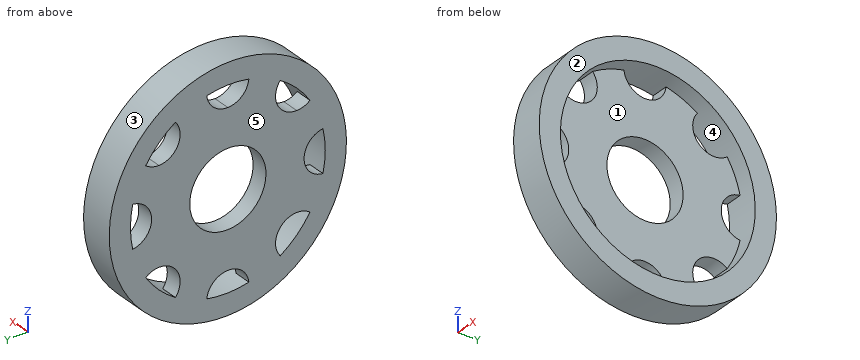
from build123d import *

# Parameters (mm, degrees)
ESBO_O1_R                = 4.5
RESSALTO_EXTRUS_O1_DEPTH = 2
ESBO_O2_R                = 14
ESBO_O2_R_2              = 11.5
RESSALTO_EXTRUS_O2_DEPTH = 2


with BuildPart() as part:
    # Esboço1 → Ressalto-extrusão1 (new body)
    with BuildSketch(Plane(origin=(0, 0, 0), x_dir=(0, 0, -1), z_dir=(1, 0, 0))):
        with BuildLine():
            ThreePointArc((11.22826087, -2.485187688), (9, 0), (11.22826087, 2.485187688))
            ThreePointArc((11.22826087, 2.485187688), (10.624614624, 4.400859472), (9.696872469, 6.182286335))
            ThreePointArc((9.696872469, 6.182286335), (6.363961031, 6.363961031), (6.182286335, 9.696872469))
            ThreePointArc((6.182286335, 9.696872469), (4.400859472, 10.624614624), (2.485187688, 11.22826087))
            ThreePointArc((2.485187688, 11.22826087), (0, 9), (-2.485187688, 11.22826087))
            ThreePointArc((-2.485187688, 11.22826087), (-4.400859472, 10.624614624), (-6.182286335, 9.696872469))
            ThreePointArc((-6.182286335, 9.696872469), (-5.773380668, 8.961304948), (-5.631727984, 8.131727984))
            ThreePointArc((-5.631727984, 8.131727984), (-7.050724101, 5.877525108), (-9.696872469, 6.182286335))
            ThreePointArc((-9.696872469, 6.182286335), (-10.624614624, 4.400859472), (-11.22826087, 2.485187688))
            ThreePointArc((-11.22826087, 2.485187688), (-9.638636545, 1.668929623), (-9, 0))
            ThreePointArc((-9, 0), (-9.638636545, -1.668929623), (-11.22826087, -2.485187688))
            ThreePointArc((-11.22826087, -2.485187688), (-10.624614624, -4.400859472), (-9.696872469, -6.182286335))
            ThreePointArc((-9.696872469, -6.182286335), (-7.050724101, -5.877525108), (-5.631727984, -8.131727984))
            ThreePointArc((-5.631727984, -8.131727984), (-5.773380668, -8.961304948), (-6.182286335, -9.696872469))
            ThreePointArc((-6.182286335, -9.696872469), (-4.400859472, -10.624614624), (-2.485187688, -11.22826087))
            ThreePointArc((-2.485187688, -11.22826087), (0, -9), (2.485187688, -11.22826087))
            ThreePointArc((2.485187688, -11.22826087), (4.400859472, -10.624614624), (6.182286335, -9.696872469))
            ThreePointArc((6.182286335, -9.696872469), (6.363961031, -6.363961031), (9.696872469, -6.182286335))
            ThreePointArc((9.696872469, -6.182286335), (10.624614624, -4.400859472), (11.22826087, -2.485187688))
        make_face()
        Circle(ESBO_O1_R, mode=Mode.SUBTRACT)
    extrude(amount=RESSALTO_EXTRUS_O1_DEPTH)

    # Esboço2 → Ressalto-extrusão2 (add, symmetric)
    with BuildSketch(Plane(origin=(2, 0, 0), x_dir=(0, 0, -1), z_dir=(1, 0, 0))):
        Circle(ESBO_O2_R)
        with Locations(Location((0, 0, 0), (0, 0, 167.519737803))):
            Circle(ESBO_O2_R_2, mode=Mode.SUBTRACT)
    extrude(amount=RESSALTO_EXTRUS_O2_DEPTH, both=True)


solid = part.part
Read the model definition and answer for the solid it produces. Units are mm, in the model's axes. Face numbers are marked on the shaded views. A direction names the side the tool comes from. Round coordinates to 2 decimals unless told otherwise and drop trailing zeros. Order: outer loops, then holes, each group sorted by start corner. A loop starts at its lowest first (then second) coordinate and runs counter-clockwise, first axis right, second up. Notation, with made-up numbers: (61.5, 37) - (74.5, 37) arc R24 cw to (74.5, 72) - close; hole circle Ø9 at (50, 11.25). An arc over 180 degrees is marked (long way). Use one line per item in the form item = value. Start each with the question number.
(1) Find the intervals of material crossed by line 1 along Z through (x, y) = (1.45, 6.75); line 2 along Y through (x, z) = (0.5, -2); line 3 along Y through (x, z) = (2.75, 2), in increasing order. Write a range as from..to.
(2) For the marked faces 1 and 2, determine the directions among +Z, -Z, +X, -X, +Y, -Y from which every point of the face is accessible in a straight line to the end or side of a thin tool.
(3) The part is cut by section A-A (z = 0). Give the vertices of the cut face in (x, y).
(4) The part is cut by section C-C (x = 2.9). Give the vertices of the cut face in (y, z).
(5) The part is cut by section B-B (y = 5.25). Give the vertices of the cut face in (x, z).
(6) Flat-ended cylindrical pins translate along their axes: pin 1 Ø2 at (x, y) = (3, -10.5) entering from +Z; pin 2 Ø2 at (x, z) = (2, -7) entering from +Y; pin 3 Ø1.5 at (x, y) = (1.5, -4) entering from -Z; pin 4 Ø4 at (y, z) = (-7, 4.5) entering from -X. Find the tip coordinate at first contact, or state that the pin passes through.
(7) Determine the mould class of the marked faces 3, 4 and 5 for opening direction Y: +Y half, -Y half, draft (parallel to the pull), parting line (faces both ways), or undercut.
(8) The part is cut by section D-D (y = -12). Give the vertices of the cut face in (x, z).
Checked values:
q1.line_1 = -12.27..-9.31, -6.05..6.05, 9.31..12.27
q1.line_2 = -13.86..-11.32, -10..-4.03, 4.03..10, 11.32..13.86
q1.line_3 = -13.86..-11.32, 11.32..13.86
q2.face_1 = +X
q2.face_2 = +Z, -Z, +X, +Y, -Y
q3.outline = (0, -14) - (4, -14) - (4, -11.5) - (0, -11.5) - close; (0, -9) - (2, -9) - (2, -4.5) - (0, -4.5) - close; (0, 4.5) - (2, 4.5) - (2, 9) - (0, 9) - close; (0, 11.5) - (4, 11.5) - (4, 14) - (0, 14) - close
q4.outline = circle Ø28 at (0, 0); hole circle Ø23 at (0, 0)
q5.outline = (0, -12.98) - (4, -12.98) - (4, -10.23) - (2, -10.23) - (2, 10.23) - (4, 10.23) - (4, 12.98) - (0, 12.98) - close
q6.pin_1 = 10.28
q6.pin_2 = 12.65
q6.pin_3 = -13.62
q6.pin_4 = 0
q7.face_3 = parting line
q7.face_4 = undercut
q7.face_5 = draft
q8.outline = (0, -7.21) - (4, -7.21) - (4, 7.21) - (0, 7.21) - close
